Autodesk Inventor part; units mm, degrees
ref_plane "Start Plane" through (0, 0, -10) normal (0, 0, 1) x (1, 0, 0)
ref_plane "End Plane" through (0, 0, 80) normal (0, 0, 1) x (1, 0, 0)
ref_plane "Work Plane4" through (0, 10, -10) normal (0, -0.7071, -0.7071) x (1, 0, 0)
ref_plane "Start Plane" through (0, 0, -10) normal (0, 0, 1) x (1, 0, 0)
ref_plane "End Plane" through (0, 0, 80) normal (0, 0, 1) x (1, 0, 0)
sketch "Sketch" plane through (0, 0, 0) normal (0, 0, 1) x (1, 0, 0)
  line L0 (-10, -6) -> (-10, 6)
  line L1 (-6, 10) -> (6, 10)
  line L2 (10, 6) -> (10, -6)
  line L3 (6, -10) -> (-6, -10)
  arc A0 (-10, -6) -> (-6, -10) centre (-6, -6) ccw
  arc A1 (10, 6) -> (6, 10) centre (6, 6) ccw
  arc A2 (-6, 10) -> (-10, 6) centre (-6, 6) ccw
  arc A3 (6, -10) -> (10, -6) centre (6, -6) ccw
  arc A4 (-6, 8) -> (-8, 6) centre (-6, 6) ccw
  line L4 (-6, 8) -> (6, 8)
  arc A5 (8, 6) -> (6, 8) centre (6, 6) ccw
  line L5 (8, 6) -> (8, -6)
  arc A6 (6, -8) -> (8, -6) centre (6, -6) ccw
  line L6 (6, -8) -> (-6, -8)
  arc A7 (-8, -6) -> (-6, -8) centre (-6, -6) ccw
  line L7 (-8, -6) -> (-8, 6)
  line L8 (0, 15.1598) -> (0, -15.1598) construction
  line L9 (-15.1598, 0) -> (15.1598, 0) construction
  dimension "d7" = 4
  dimension "d9" = 20
  dimension "d11" = 20
  dimension "d12" = 2
  dimension "d15" = 10
  dimension "d16" = 10
extrude "Body" add sketch "Sketch" along normal up to surface (90 mm away) from surface at -10
sketch "Sketch3" plane through (0, 0, 0) normal (0, 0, 1) x (1, 0, 0)
  line L0 (0, 0) -> (10, 0)
ref_plane "Work Plane3" through (0, 0, 0) normal (0, -1, 0) x (1, 0, 0)
ref_plane "Work Plane4" through (0, 10, -10) normal (0, -0.7071, -0.7071) x (1, 0, 0)
split "Split1" plane through (0, 10, -10) removes the side toward (0, -0.7071, -0.7071)
sketch "Sketch4" plane through (0, 0, 0) normal (0, -1, 0) x (1, 0, 0)
  line L0 (-2, -10) -> (12, -10)
  line L1 (-2, 80) -> (12, 80)
  dimension "d18" = 90
equation "\"d7\" = G_IR"
equation "\"d9\" = G_W"
equation "\"d11\" = G_H"
equation "\"d12\" = G_T"
equation "\"d15\" = 0.5 * d9"
equation "\"d16\" = 0.5 * d11"
equation "\"d3\" = G_L"
equation "\"G_W\" = 20"
equation "\"G_H\" = 20"
equation "\"G_T\" = 2"
equation "\"G_IR\" = 4"
equation "\"G_L\" = d18"
equation "\"G_OFFSET_END\" = 0"
properties part number "ISO 10799-2 - 20x20x2 - 90" material "Steel"
Part model, mm, in its own coordinate system. A direction names the side the tool comes from. Round coordinates to 2 decimals unless told otherwise and drop trailing zeros. Loops run counter-clockwise (first coordinate to the right, second up) from the corner with the lowest first, then second, coordinate; pieces in that order, holes last. Notation, with made-up numbers: (-23.75, 44.5) -> (0.25, 44.5) arc R22 cw to (0.25, 62.5) -> close; hole circle Ø9 at (1.25, 19.5). An arc over 180 degrees is marked (long way). Use CSV: the item, a comma, the result in double quotes. Start each with the question number.
1) Drop a flat-ended pin along its axis: P1, Ø4, axis at x = 7.5, z = 13, coming from the -Y side. Give the stop position or say it passes through.
2) Cut at C-C, the plane x = -4.25. Write the cut outline in (y, z), plus the area to 3 significant figures.
3) Cut at A-A, the plane y = -1.5. Write the cut outline in (x, z), plus the area to 3 significant figures.
4) Cut at B-B, the plane z = 21. Write the cut outline in (x, y).
5) Wall check: L1, parallel to Y at x = -2, z = 38.5; L2, parallel to X at y = -6.25, z = 20.5; L3, parallel to Y at x = -1, z = 0.5. Give the ranges that are in metal, low to high. Write a range as [from, to].
6) Cut at D-D, the plane z = 1. Write the cut outline in (x, y).
7) Pull direction X, two halves, no side cores. Call faces 1 (the flat face through (-8.2, 0, 0)), 2 (the flat face through (-10, 0, 36)), 3 (the cylindrical face through (7.43, -7.4, 42.48)): +X half, -X half, draft (parallel to the pull), parting line (faces both ways), or undercut.
8) Which spindle directions (+Z, -Z, +X, -X, +Y, -Y) get a long thin tool onto all of the face, cutting with end or side? Do faces 4 (the flat face through (0, -8, 43)), 5 (the flat face through (10, 0, 36)). Say none if no direction does.
Determined:
1,P1,"stops at y = -10"
2,outline,"(-10, 10) -> (-8, 8) -> (-8, 80) -> (-10, 80) -> close; (8, -8) -> (10, -10) -> (10, 80) -> (8, 80) -> close"
2,area,"320 mm2"
3,outline,"(-10, 1.5) -> (-8, 1.5) -> (-8, 80) -> (-10, 80) -> close; (8, 1.5) -> (10, 1.5) -> (10, 80) -> (8, 80) -> close"
3,area,"314 mm2"
4,outline,"(-10, -6) arc R4 ccw to (-6, -10) -> (6, -10) arc R4 ccw to (10, -6) -> (10, 6) arc R4 ccw to (6, 10) -> (-6, 10) arc R4 ccw to (-10, 6) -> close; hole (-8, -6) arc R2 ccw to (-6, -8) -> (6, -8) arc R2 ccw to (8, -6) -> (8, 6) arc R2 ccw to (6, 8) -> (-6, 8) arc R2 ccw to (-8, 6) -> close"
5,L1,"y = [-10, -8], [8, 10]"
5,L2,"x = [-9.99, -7.98], [7.98, 9.99]"
5,L3,"y = [8, 10]"
6,outline,"(-10, -1) -> (-8, -1) -> (-8, 6) arc R2 cw to (-6, 8) -> (6, 8) arc R2 cw to (8, 6) -> (8, -1) -> (10, -1) -> (10, 6) arc R4 ccw to (6, 10) -> (-6, 10) arc R4 ccw to (-10, 6) -> close"
7,face 1,"draft"
7,face 2,"-X half"
7,face 3,"undercut"
8,face 4,"+Z, -Z"
8,face 5,"+Z, -Z, +X, +Y, -Y"
